```python
from build123d import *

# Parameters (mm, degrees)
BOSS_EXTRUDE1_DEPTH = 9.525
CUT_EXTRUDE1_DEPTH  = 10.525
SKETCH3_R           = 6.35
SKETCH3_R_2         = 1.5875
CUT_EXTRUDE2_DEPTH  = 10.525
SKETCH4_R           = 2.4638
CUT_EXTRUDE3_DEPTH  = 10.525


with BuildPart() as part:
    # Sketch1 → Boss-Extrude1 (new body)
    with BuildSketch(Plane(origin=(0, 0, 0), x_dir=(0, 0, -1), z_dir=(1, 0, 0))):
        Polygon((0, 0), (275.149828585, 365.136155194), (336.005854451, 319.277850429), (95.412737152, 0), align=None)
    extrude(amount=BOSS_EXTRUDE1_DEPTH)

    # Sketch2 → Cut-Extrude1 (cut, through all)
    with BuildSketch(Plane(origin=(9.525, 0, 0), x_dir=(0, 0, -1), z_dir=(1, 0, 0))):
        with BuildLine():
            Line((335.050473101, 318.010016557), (314.765131146, 333.296118145))
            ThreePointArc((314.765131146, 333.296118145), (313.753290935, 334.591214557), (313.524559813, 336.218721055))
            Line((313.524559813, 336.218721055), (336.005854451, 319.277850429))
            Line((336.005854451, 319.277850429), (335.050473101, 318.010016557))
        make_face()
    extrude(amount=-CUT_EXTRUDE1_DEPTH, mode=Mode.SUBTRACT)

    # Sketch3 → Cut-Extrude2 (cut, through all)
    with BuildSketch(Plane(origin=(9.525, 0, 0), x_dir=(0, 0, -1), z_dir=(1, 0, 0))):
        with Locations((187.569137258, 185.604162917)):
            Circle(SKETCH3_R)
        with Locations((195.663087406, 170.599745201)):
            Circle(SKETCH3_R_2)
        with Locations((181.400785207, 164.545757096)):
            Circle(SKETCH3_R_2)
        with Locations((169.026726614, 173.870279065)):
            Circle(SKETCH3_R_2)
        with Locations((170.914970221, 189.248789139)):
            Circle(SKETCH3_R_2)
        with Locations((185.17727242, 195.302777243)):
            Circle(SKETCH3_R_2)
        with Locations((197.551331013, 185.978255275)):
            Circle(SKETCH3_R_2)
    extrude(amount=-CUT_EXTRUDE2_DEPTH, mode=Mode.SUBTRACT)

    # Sketch4 → Cut-Extrude3 (cut, through all)
    with BuildSketch(Plane(origin=(9.525, 0, 0), x_dir=(0, 0, -1), z_dir=(1, 0, 0))):
        with Locations((285.346343492, 336.461727915)):
            Circle(SKETCH4_R)
        with Locations((276.786126603, 325.10193642)):
            Circle(SKETCH4_R)
        with Locations((39.6875, 30.988)):
            Circle(SKETCH4_R)
        with Locations((39.6875, 16.764)):
            Circle(SKETCH4_R)
        with Locations((82.55, 30.988)):
            Circle(SKETCH4_R)
        with Locations((82.55, 16.764)):
            Circle(SKETCH4_R)
    extrude(amount=-CUT_EXTRUDE3_DEPTH, mode=Mode.SUBTRACT)


solid = part.part
```
The listing builds one solid part. Answer for the finished solid, in the listing's coordinates (mm). Coordinates: 2 decimals unless noted, no trailing zeros. Loops run counter-clockwise (first coordinate to the right, second up) from the corner with the lowest first, then second, coordinate; pieces in that order, holes last. Notation, with made-up numbers: M -23,50 L 10,50 A21 cw 10,87 Z; hole C 74.5,-21.5 d10. An arc over 180 degrees is marked long. Answer as a JSON object with one key per item and string values. Group by question number.
Item 1: Each of these flat-tipped pins is pushed along its axis until it touches: P1, Ø4, axis at y = 336.46, z = -285.35, coming from the +X side; P2, Ø3, axis at x = 6, z = -234.5, coming from the +Y side; P3, Ø5, axis at x = 7, z = -208.5, coming from the +Y side; P4, Ø1, axis at x = 3, y = 157, coming from the -Z side. Where does it stop, or does it pass through?
Item 2: Determine the mould class of faces 1 (the face through (4.83, 181.74, -182.53)), 2 (the face through (0, 170, -181)), 3 (the face through (4.696, 180.012, -135.649)) for opening direction Z: +Z half, -Z half, draft (parallel to the pull), parting line (faces both ways), or undercut.
Item 3: Section B-B (z = -56) is taken. Write down the section's boundary in (x, y) (3 decimals).
Item 4: Section A-A (x = 4) is taken. Give the number of separate pieces and of enclosed holes in the cut face, and give its area (3 significant figures).
Item 5: Section C-C (y = 45) is taken. Write down the section's boundary in (x, z) (3 decimals).
Item 6: Consider L1, parallel to Y at x = 4.25, z = -170; L2, parallel to Y at x = 6.75, z = -82.55; L3, parallel to Y at x = 2.5, z = -279. Determine where each line is inside the solid, lowest interval first.
Solved:
{
 "1": {"P1": "passes through", "P2": "stops at y = 313.18", "P3": "stops at y = 280.01", "P4": "stops at z = -214.1"},
 "2": {"face 1": "undercut", "face 2": "draft", "face 3": "+Z half"},
 "3": {"outline": "M 0,0 L 9.525,0 L 9.525,74.315 L 0,74.315 Z"},
 "4": {"separate pieces": "1", "enclosed holes": "13", "area": "32,300 mm2"},
 "5": {"outline": "M 0,-129.323 L 9.525,-129.323 L 9.525,-33.91 L 0,-33.91 Z"},
 "6": {"L1": "y = 98.98 to 172.62, 175.12 to 187.95, 190.55 to 225.6", "L2": "y = 0 to 14.3, 19.23 to 28.52, 33.45 to 109.55", "L3": "y = 243.63 to 324.02, 326.18 to 362.23"}
}
